Answer from the drawing. Dimensions are ordinates in mm from the lowest x, y and z of the part. A direction names the side the tool comes from. Give positions to 0.01 mm unless a question says otherwise; leave off trailing zeros. Order: outer loops, then holes, each group sorted by start corner. A loop starts at its lowest first (then second) coordinate and runs counter-clockwise, first axis right, second up.
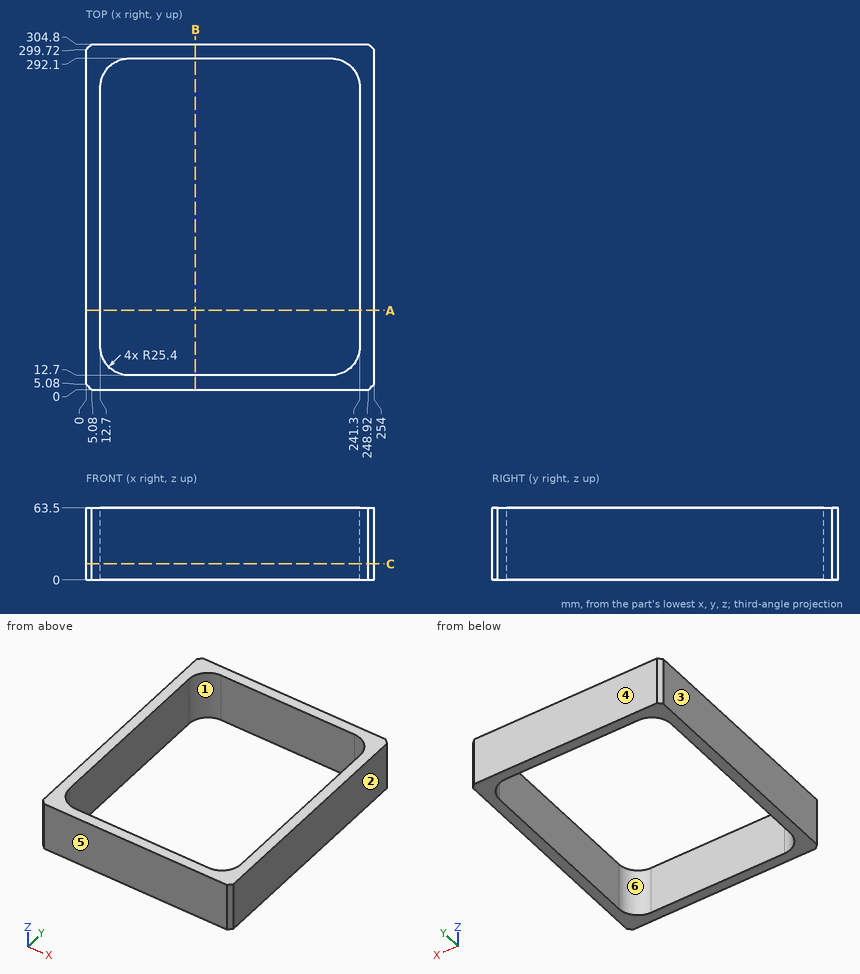
1) The part is cut by section B-B on x = 96.5. Determine the outline of the cut face in (y, z), and give its area (3 significant figures).
Final values:
outline: (0, 0) - (12.7, 0) - (12.7, 63.5) - (0, 63.5) - close; (292.1, 0) - (304.8, 0) - (304.8, 63.5) - (292.1, 63.5) - close
area: 1,610 mm2
2) The part is cut by section A-A on y = 70. Determine the outline of the cut face in (x, z), and give its area (3 significant figures).
Final values:
outline: (0, 0) - (12.7, 0) - (12.7, 63.5) - (0, 63.5) - close; (241.3, 0) - (254, 0) - (254, 63.5) - (241.3, 63.5) - close
area: 1,610 mm2
3) For a pull along X with two mould halves and no side action, classify the marked faces 1, 2, 3 and 4 as released by +X, released by -X, zero draft, split by the parting line, or undercut.
Final values:
face 1: undercut
face 2: released by +X
face 3: released by -X
face 4: zero draft
4) Consider L1, parallel to Y at x = 194.5, z = 26; L2, parallel to X at y = 55.5, z = 15; L3, parallel to Y at x = 219, z = 54. Determine where each line is inside the solid, lowest interval first.
Final values:
L1: y = 0 to 12.7, 292.1 to 304.8
L2: x = 0 to 12.7, 241.3 to 254
L3: y = 0 to 12.89, 291.91 to 304.8
5) A tool of negligible diameter and unlimited length cuts with its end or side. For the marked faces 5 and 6, from which of +Z, -Z, +X, -X, +Y, -Y can it reach the whole face along a straight path? Write none if from no direction.
Final values:
face 5: +Z, -Z, +X, -X, -Y
face 6: +Z, -Z
6) The part is cut by section C-C on z = 14. Determine the outline of the cut face in (x, y).
Final values:
outline: (0, 5.08) - (5.08, 0) - (248.92, 0) - (254, 5.08) - (254, 299.72) - (248.92, 304.8) - (5.08, 304.8) - (0, 299.72) - close; hole (12.7, 38.1) arc R25.4 ccw to (38.1, 12.7) - (215.9, 12.7) arc R25.4 ccw to (241.3, 38.1) - (241.3, 266.7) arc R25.4 ccw to (215.9, 292.1) - (38.1, 292.1) arc R25.4 ccw to (12.7, 266.7) - close
